Part model, mm, in its own coordinate system. Face numbers are marked on the shaded views. Coordinates: 2 decimals unless noted, no trailing zeros. Loops run counter-clockwise (first coordinate to the right, second up) from the corner with the lowest first, then second, coordinate; pieces in that order, holes last. Notation, with made-up numbers: (38.25, 22) -> (87.25, 22) arc R35 cw to (87.25, 55) -> close; hole circle Ø8 at (8.25, 64). An arc over 180 degrees is marked (long way). One line per question, with ' | ' between items. Start each with the question number.
1) Cut at B-B (x = -1). List the corners of the cut face in (y, z).
2) Cut at C-C (y = 0.55). List the corners of the cut face in (x, z) (1 decimal).
3) Cut at D-D (x = 11.5). List the corners of the cut face in (y, z), plus the area to 3 significant figures.
4) Cut at A-A (z = 16). List the corners of the cut face in (x, y), plus the area to 3 significant figures.
5) Two-plate mould, pull along Y, no slides. Class the marked faces 1 and 2: released by +Y, released by -Y, zero draft, split by the parting line, or undercut.
6) Probe L1, parallel to X at y = 0.4, z = 29 (3 decimals); L2, parallel to X at y = 0.5, z = 0; L3, parallel to X at y = 0.5, z = 14. List the from-to ranges inside material, lowest first. Write a range as from..to.
7) Drop flat-ended pins along their axis: pin 1 (0.8 mm diameter, centred on x = -11.5, z = 28.5, fed in from +Y); pin 2 (1.6 mm diameter, centred on x = 11.5, z = 29, fed in from +Y). Give the stop position or say it passes through.
Autodesk Inventor part; units mm, degrees
ref_plane "YZ Plane" through (0, 0, 0) normal (1, 0, 0) x (0, 1, 0)
ref_plane "XZ Plane" through (0, 0, 0) normal (0, 1, 0) x (-1, 0, 0)
ref_plane "XY Plane" through (0, 0, 0) normal (0, 0, 1) x (1, 0, 0)
sketch "スケッチ1" plane through (0, 0, 0) normal (0, 1, 0) x (-1, 0, 0)
  circle A0 centre (11.5, 0) radius 0.85
  circle A1 centre (11.5, 29) radius 0.85
  line L0 (0, -11.6446) -> (0, 36.0381)
  arc A2 (12.3932, 27.0169) -> (9.325, 29) centre (11.5, 29) ccw
  arc A3 (12.6962, -1.8165) -> (12.3932, 1.9831) centre (11.5, 0) ccw
  circle A4 centre (0, 0) radius 5
  line L1 (4, 23.5) -> (4, -3)
  line L2 (4, -3) -> (1.6185, -4.5259)
  line L3 (12.6962, -1.8165) -> (4.675, -7.0989)
  arc A5 (0, -8.5) -> (4.675, -7.0989) centre (0, 0) ccw
  circle A6 centre (0, -2) radius 3
  line L4 (4, 23.5) -> (0, 23.5)
  line L5 (14.3325, 28.15) -> (9.1092, 28.15)
  line L6 (-4, 23.5) -> (-4, -3)
  line L7 (-4, -3) -> (-1.6185, -4.5259)
  line L8 (-4, 23.5) -> (0, 23.5)
  line L9 (6.5, 11.1009) -> (6.5, 17.8991)
  arc A7 (6.325, 26) -> (9.325, 29) centre (6.325, 29) ccw
  line L10 (6.325, 26) -> (0, 26)
  arc A8 (12.3932, 27.0169) -> (6.5, 17.8991) centre (16.5, 17.8991) ccw
  arc A9 (6.5, 11.1009) -> (12.3932, 1.9831) centre (16.5, 11.1009) ccw
  circle A10 centre (11.5, 0) radius 1.175
  circle A11 centre (11.5, 29) radius 1.175
  point P0 (0, 30.9357)
  point P1 (4, 3)
  point P2 (0, 26.5)
  point P3 (0, -5)
  point P4 (-1.6185, -4.5259)
  point P5 (0, 1)
  point P6 (-4, 3)
  point P7 (0, -5)
  point P8 (3.4728, -6.6475)
  point P9 (0, 5)
  point P10 (0, -5)
  point P11 (2.7322, -4.1875)
  point P12 (-4, -3)
  dimension "d7" = 10
  dimension "d2" = 29
  dimension "d18" = 8.5
  dimension "d24" = 1.7
  dimension "d25" = 2
  dimension "d39" = 8
  dimension "d41" = 2.5
  dimension "d43" = 2.5
  dimension "d44" = 10
  dimension "d45" = 23
  dimension "d47" = 3
  dimension "d48" = 2.35
  dimension "d49" = 1
  dimension "d50" = 1
extrude "押し出し1" add sketch "スケッチ1" along normal blind 0.75 contours L5 A11 | L5 A11 | A11 L5 A7 A2 | L5 A2 A8 L9 A9 A3 L3 A5 L0 A4 L1 L4 L10 A7 A11 | A4 L1 | A6 L2 A4 | A10
sketch "スケッチ2" plane through (0, 0.75, 0) normal (0, 1, 0) x (1, 0, 0)
  circle A0 centre (-11.5, 0) radius 1.3
  circle A1 centre (-11.5, 0) radius 0.85
  circle A2 centre (-11.5, -29) radius 0.85
  circle A3 centre (-11.5, -29) radius 0.85
  circle A4 centre (-11.5, -29) radius 1.3
  point P0 (0, 0)
  dimension "d51" = 2.6
extrude "押し出し2" cut sketch "スケッチ2" against normal blind 0.5
mirror "ミラー2" about plane through (0, 0, 26) normal (1, 0, 0) of "押し出し1", "押し出し2"
properties part number "Skirt"
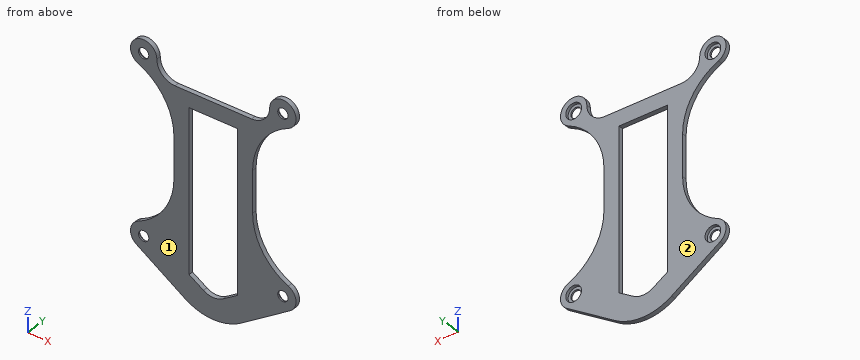
Reported:
1) outline: (0, -8.44) -> (0.75, -8.44) -> (0.75, -4.83) -> (0, -4.83) -> close; (0, 23.5) -> (0.75, 23.5) -> (0.75, 26) -> (0, 26) -> close
2) outline: (-12.7, -1.8) -> (-4.7, -7.1) arc R8.5 ccw to (0, -8.5) arc R8.5 ccw to (4.7, -7.1) -> (12.7, -1.8) arc R2.2 ccw to (12.4, 2) arc R10 cw to (6.5, 11.1) -> (6.5, 17.9) arc R10 cw to (12.4, 27) arc R2.2 ccw (long way) to (9.3, 29) arc R3 cw to (6.3, 26) -> (-6.3, 26) arc R3 cw to (-9.3, 29) arc R2.2 ccw (long way) to (-12.4, 27) arc R10 cw to (-6.5, 17.9) -> (-6.5, 11.1) arc R10 cw to (-12.4, 2) arc R2.2 ccw to start; hole circle Ø2.6 at (-11.5, 0); hole circle Ø2.6 at (-11.5, 29); hole (-4, -3) -> (-1.6, -4.5) arc R3 ccw to (1.6, -4.5) -> (4, -3) -> (4, 23.5) -> (-4, 23.5) -> close; hole circle Ø2.6 at (11.5, 0); hole circle Ø2.6 at (11.5, 29)
3) outline: (0, -2.6) -> (0.75, -2.6) -> (0.75, -1.3) -> (0.25, -1.3) -> (0.25, -0.85) -> (0, -0.85) -> close; (0, 0.85) -> (0.25, 0.85) -> (0.25, 1.3) -> (0.75, 1.3) -> (0.75, 2.44) -> (0, 2.44) -> close; (0, 26.56) -> (0.75, 26.56) -> (0.75, 27.7) -> (0.25, 27.7) -> (0.25, 28.15) -> (0, 28.15) -> close; (0, 29.85) -> (0.25, 29.85) -> (0.25, 30.3) -> (0.75, 30.3) -> (0.75, 31.17) -> (0, 31.17) -> close | area: 3.80 mm²
4) outline: (-6.5, 0) -> (-4, 0) -> (-4, 0.75) -> (-6.5, 0.75) -> close; (4, 0) -> (6.5, 0) -> (6.5, 0.75) -> (4, 0.75) -> close | area: 3.75 mm²
5) face 1: released by -Y | face 2: released by +Y
6) L1: x = -13.675..-12.8, -10.2..-9.325, 9.325..10.2, 12.8..13.675 | L2: x = -13.67..-12.8, -10.2..-4, 4..10.2, 12.8..13.67 | L3: x = -6.5..-4, 4..6.5
7) pin 1: stops at y = 0.25 | pin 2: passes through
